Can you work these out from the model? Positions are in its coordinate system, mm. Coordinates: 2 decimals unless noted, no trailing zeros. Write each loop counter-clockwise with the first axis right and the second up, starting at its lowest first coordinate (ties: lowest second). Pieces come first, ordered by that corner, then holes. Notation, with made-up numbers: M -22,71.25 L -15,71.25 A21 ccw -15,91.25 Z; hole C 7,-26.75 d5. An arc over 180 degrees is marked long. Use one line per item in the form item = value. Start each with the question number.
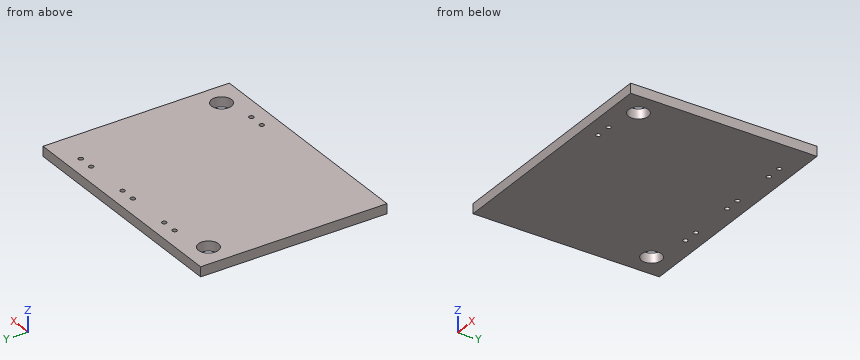
```python
from build123d import *

# Parameters (mm, degrees)
SKETCH1_W                 = 38.735
SKETCH1_H                 = 30.48
BOSS_EXTRUDE1_DEPTH       = 0.8
F_4_CLEARANCE_HOLE1_D     = 3.2639
F_4_CLEARANCE_HOLE1_DEPTH = 10.922
F_4_CLEARANCE_HOLE1_TIP   = 0.980574487
SKETCH6_R                 = 0.381
CUT_EXTRUDE1_DEPTH        = 2.6


with BuildPart() as part:
    # Sketch1 → Boss-Extrude1 (new body, symmetric)
    with BuildSketch(Plane.XY):
        Rectangle(SKETCH1_W, SKETCH1_H)
    extrude(amount=BOSS_EXTRUDE1_DEPTH, both=True)

    # #4 Clearance Hole1
    with Locations(Plane.XY.offset(0.8)):
        with Locations((-15.5575, 11.43), (15.5575, -11.43)):
            Hole(F_4_CLEARANCE_HOLE1_D / 2, depth=F_4_CLEARANCE_HOLE1_DEPTH)
            with Locations((0, 0, -(F_4_CLEARANCE_HOLE1_DEPTH + F_4_CLEARANCE_HOLE1_TIP / 2))):  # 118° drill point
                Cone(0, F_4_CLEARANCE_HOLE1_D / 2, F_4_CLEARANCE_HOLE1_TIP, mode=Mode.SUBTRACT)

    # Sketch6 → Cut-Extrude1 (cut, through all)
    with BuildSketch(Plane.XY.offset(0.8)):
        with Locations((-9.289404292, 12.804978229)):
            Circle(SKETCH6_R)
        with Locations((-6.749404292, 12.804978229)):
            Circle(SKETCH6_R)
        with Locations((0.943821165, 12.804978229)):
            Circle(SKETCH6_R)
        with Locations((3.483821165, 12.804978229)):
            Circle(SKETCH6_R)
        with Locations((11.19802304, 12.804978229)):
            Circle(SKETCH6_R)
        with Locations((13.73802304, 12.804978229)):
            Circle(SKETCH6_R)
        with Locations((7.59553263, -12.709329553)):
            Circle(SKETCH6_R)
        with Locations((10.13553263, -12.709329553)):
            Circle(SKETCH6_R)
    extrude(amount=-CUT_EXTRUDE1_DEPTH, mode=Mode.SUBTRACT)


solid = part.part
```
1) Suppose I cut it at B-B on z = -0.1. State how many separate pieces and enclosed holes the cut face has, and give its area (3 significant figures).
2) Will this pin go through, and if not, where does the flat tip stop? pin 1 Ø3 at (x, y) = (-15.56, 11.43) entering from +Z.
3) Suppose I cut it at A-A on y = 11.43. Please give me the cut outline in (x, z).
4) Please list where these lines run through material, in increasing order: line 1 (X direction, y = 12, z = -0.5); line 2 (Y direction, x = -7, z = -0.3).
Computed values:
q1.separate_pieces = 1
q1.enclosed_holes = 10
q1.area = 1,160 mm²
q2.pin_1 = through
q3.outline = M -19.37,-0.8 L -17.19,-0.8 L -17.19,0.8 L -19.37,0.8 Z; M -13.93,-0.8 L 19.37,-0.8 L 19.37,0.8 L -13.93,0.8 Z
q4.line_1 = -19.37 to -17.09, -14.03 to 19.37
q4.line_2 = -15.24 to 12.52, 13.09 to 15.24
